```python
from build123d import *

# Parameters (mm, degrees)
F1_DEPTH = 40
F4_R     = 4
F6_R     = 2
F8_DEPTH = 6.281


with BuildPart() as f1:
    # F0 (on Top) → F1 (new body)
    with BuildSketch(Plane.XY):
        Polygon((0, 3.62576), (-3.14, 1.81288), (-3.14, -1.81288), (0, -3.62576), (3.14, -1.81288), (3.14, 1.81288), align=None)
    extrude(amount=F1_DEPTH)

    # F5: sweep along a path in F3
    with BuildLine(Plane.XY.offset(10.5)) as f5_path:
        CenterArc((0, 0), 6.75, 0, 360)
    # F4 (on Front) → F5 (sweep, cut)
    with BuildSketch(Plane.XZ):
        with Locations((-6.75, 10.5)):
            Circle(F4_R)
    sweep(path=f5_path.line, mode=Mode.SUBTRACT)

    # F6
    f6_edges = [f1.edges().sort_by_distance(p)[0] for p in [
        (1.57, -2.71932, 40),
        (-1.57, -2.71932, 40),
        (3.14, 0, 40),
        (-1.57, 2.71932, 40),
        (-3.14, 0, 40),
        (1.57, 2.71932, 40),
    ]]
    fillet(f6_edges, radius=F6_R)

    # F7 (on face) → F8 (cut, through all)
    with BuildSketch(Plane(origin=(-3.14, 0, 0), x_dir=(0, -1, 0), z_dir=(-1, 0, 0))):
        Polygon((1.81288, 31.650778), (0, 34.840249), (-1.81288, 31.650778), (-1.81288, 28.396215), (1.81288, 28.396215), align=None)
    extrude(amount=-F8_DEPTH, mode=Mode.SUBTRACT)


solid = f1.part
```
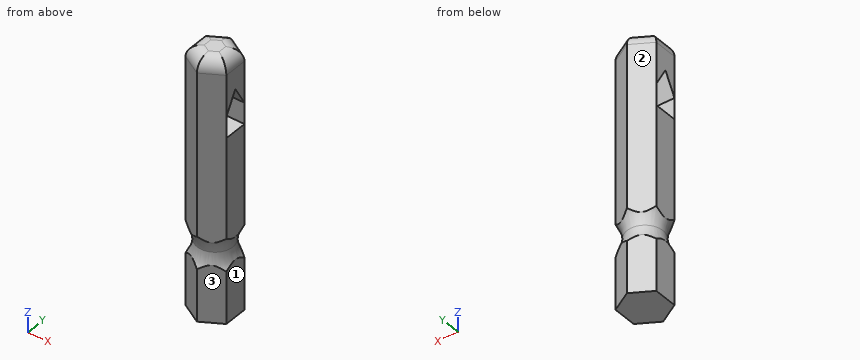
CAD build for the part. Positions are in the model's coordinates, mm. Face numbers are marked on the shaded views. Round coordinates to 2 decimals unless told otherwise and drop trailing zeros. Order: outer loops, then holes, each group sorted by start corner. A loop starts at its lowest first (then second) coordinate and runs counter-clockwise, first axis right, second up. Notation, with made-up numbers: (14, 21) - (55, 21) arc R18 cw to (55, 45) - close; hole circle Ø9 at (70, 47). An arc over 180 degrees is marked (long way). Use CSV: the item, a comma, the result in double quotes. Start each with the question number.
1) Saw through at A-A (z = 16). List the corners of the cut face in (x, y).
2) Two-plate mould, pull along Y, no slides. Class the marked faces 1, 2 and 3: pulls with the +Y half, pulls with the -Y half, needs draft (parallel to the pull), parting line crosses it, or undercut.
3) Wall check: L1, parallel to Z at x = 1.75, y = -1.75; L2, parallel to Y at x = 1, z = 7.5; L3, parallel to Z at x = 1.25, y = 1. Give the ranges that are in metal, low to high. Write a range as [from, to].
4) Saw through at B-B (z = 9.5). List the corners of the cut face in (x, y), and give its area (3 significant figures).
5) Pin check, flat tips, straight feed: pin 1 Ø1.6 at (x, z) = (-1.5, 30.5) entering from +Y; pin 2 Ø2 at (y, z) = (-2.5, 11.5) entering from +X; pin 3 Ø2.5 at (x, z) = (-1.5, 30.5) entering from -Y. Stop position of each tip, or through.
Values follow:
1,outline,"(-3.14, -1.81) - (0, -3.63) - (3.14, -1.81) - (3.14, 1.81) - (0, 3.63) - (-3.14, 1.81) - close"
2,face 1,"needs draft"
2,face 2,"pulls with the +Y half"
2,face 3,"pulls with the -Y half"
3,L1,"z = [0, 28.4], [31.76, 39.56]"
3,L2,"y = [-3.05, 3.05]"
3,L3,"z = [0, 28.4], [33.08, 39.97]"
4,outline,"circle Ø5.75 at (0, 0)"
4,area,"26.0 mm2"
5,pin 1,"stops at y = 3.22"
5,pin 2,"stops at x = 2.57"
5,pin 3,"stops at y = -3.48"
